Input: part model. Units: mm. Frame: model coordinates. A direction names the side the tool comes from. Coordinates: 2 decimals unless noted, no trailing zeros. Loops run counter-clockwise (first coordinate to the right, second up) from the corner with the lowest first, then second, coordinate; pieces in that order, holes last. Notation, with made-up numbers: M -32,-16 L 5,-16 A15 cw 5,-3 Z; hole C -38.5,37 d11. An arc over 180 degrees is marked long. Use a Markdown table: item, result. Add a question column.
1. Section B-B on z = 4. Output: boundary loops of the cut face in (x, y), then the cut area to 3 significant figures.
2. Line query: L1, parallel to X at y = -5.25, z = 4; L2, parallel to Z at x = 25, y = -11; L3, parallel to X at y = -8, z = 6.5. Output: solid intervals per line, ascending. Write a range as [from, to].
3. Section A-A on y = -12.5. Output: boundary loops of the cut face in (x, z).
4. Section D-D on y = 15.5. Output: boundary loops of the cut face in (x, z).
5. Draft query along X for faces 4 (the flat face through (-25, -17, 6)), 5 (the cylindrical face through (-26.27, -3.7, 3.03)), 6 (the flat face through (-29, -4, 4)). Return one class per face: +X half, -X half, draft (parallel to the pull), parting line (faces both ways), or undercut.
6. Pin query (flat end, axial travel): pin 1 (1 mm diameter, centred on x = 23, z = 6, fed in from +Y); pin 2 (3 mm diameter, centred on x = -25, z = 4, fed in from -Y) (3 decimals); pin 3 (3.5 mm diameter, centred on x = -19, z = 4, fed in from -Y); pin 4 (1.5 mm diameter, centred on y = 16, z = 6, fed in from +X). Return the tip coordinate at first contact, or that it passes through.
7. Set-up query: faces 1 (the flat face through (25, 9.236, 6)), 2 (the flat face through (20.9, -8, 4)), 3 (the flat face through (-25, 9.236, 6)). Return all of +Z, -Z, +X, -X, +Y, -Y with unobstructed straight access to the full face (end or side cutting, diameter ignored); none if empty.
8. Section C-C on x = -25. Output: boundary loops of the cut face in (y, z), then the cut area to 3 significant figures.
```python
from build123d import *

# Parameters (mm, degrees)
EXTRUDE_1_DEPTH          = 8
CUT_EXTRUDE_1_DEPTH      = 50.930176246
CUT_EXTRUDE_1_DEPTH_BACK = 50.930176246
SKETCH_2_R               = 1.6


with BuildPart() as part:
    # ｽｹｯﾁ1 → ﾎﾞｽ - 押し出し1 (new body)
    with BuildSketch(Plane.XY):
        with BuildLine():
            Line((-20.9, 9.236476601), (-29, 9.236476601))
            Line((-29, 9.236476601), (-29, -17))
            Line((-29, -17), (-20.9, -17))
            Line((-20.9, -17), (-20.9, 1))
            Line((-20.9, 1), (-17.821966783, 1))
            ThreePointArc((-17.821966783, 1), (0, 17.85), (17.821966783, 1))
            Line((17.821966783, 1), (20.9, 1))
            Line((20.9, 1), (20.9, -17))
            Line((20.9, -17), (29, -17))
            Line((29, -17), (29, 9.236476601))
            Line((29, 9.236476601), (20.9, 9.236476601))
            ThreePointArc((20.9, 9.236476601), (0, 22.85), (-20.9, 9.236476601))
        make_face()
    extrude(amount=EXTRUDE_1_DEPTH)

    # ｽｹｯﾁ2 → ｶｯﾄ - 押し出し1 (cut, two sides: drawn at the far end of the back side and taken through both)
    with BuildSketch(Plane.XZ.offset(17).offset(-CUT_EXTRUDE_1_DEPTH_BACK)):
        with Locations((-25, 4)):
            Circle(SKETCH_2_R)
        with Locations((25, 4)):
            Circle(SKETCH_2_R)
    extrude(amount=CUT_EXTRUDE_1_DEPTH + CUT_EXTRUDE_1_DEPTH_BACK, mode=Mode.SUBTRACT)


solid = part.part
```
Answers below:
| question | item | result |
|---|---|---|
| 1 | outline | M -29,-17 L -26.6,-17 L -26.6,9.24 L -29,9.24 Z; M -23.4,-17 L -20.9,-17 L -20.9,1 L -17.82,1 A17.85 cw 17.82,1 L 20.9,1 L 20.9,-17 L 23.4,-17 L 23.4,9.24 L 20.9,9.24 A22.85 ccw -20.9,9.24 L -23.4,9.24 Z; M 26.6,-17 L 29,-17 L 29,9.24 L 26.6,9.24 Z |
| 1 | area | 546 mm² |
| 2 | L1 | x = [-29, -26.6], [-23.4, -20.9], [20.9, 23.4], [26.6, 29] |
| 2 | L2 | z = [0, 2.4], [5.6, 8] |
| 2 | L3 | x = [-29, -20.9], [20.9, 29] |
| 3 | outline | M -29,0 L -20.9,0 L -20.9,8 L -29,8 Z; M 20.9,0 L 29,0 L 29,8 L 20.9,8 Z; hole C -25,4 d3.2; hole C 25,4 d3.2 |
| 4 | outline | M -16.79,0 L -8.85,0 L -8.85,8 L -16.79,8 Z; M 8.85,0 L 16.79,0 L 16.79,8 L 8.85,8 Z |
| 5 | face 4 | draft |
| 5 | face 5 | undercut |
| 5 | face 6 | -X half |
| 6 | pin 1 | stops at y = 9.24 |
| 6 | pin 2 | passes through |
| 6 | pin 3 | stops at y = 1 |
| 6 | pin 4 | stops at x = 17.02 |
| 7 | face 1 | +Z, -Z, +X, +Y |
| 7 | face 2 | +Z, -Z, -Y |
| 7 | face 3 | +Z, -Z, -X, +Y |
| 8 | outline | M -17,0 L 9.24,0 L 9.24,2.4 L -17,2.4 Z; M -17,5.6 L 9.24,5.6 L 9.24,8 L -17,8 Z |
| 8 | area | 126 mm² |
